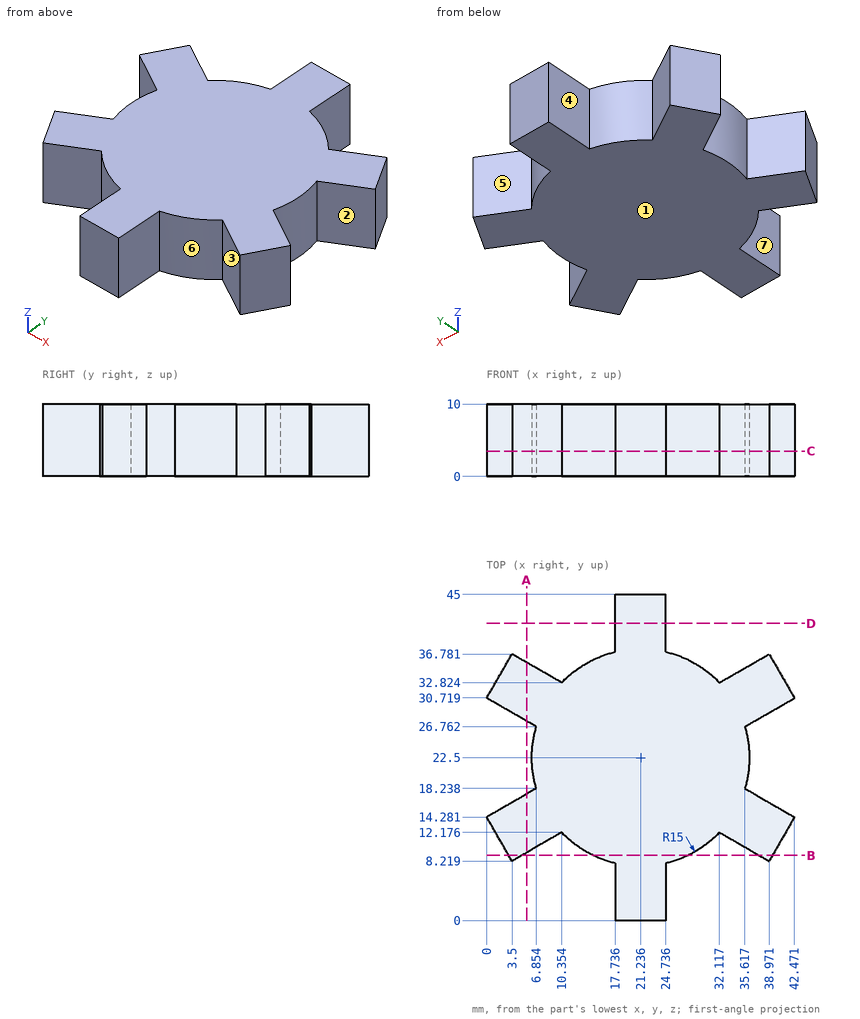
Job drawing, mm, ordinate dimensions from the low corner. One solid piece. A direction names the side the tool comes from. Coordinates: 2 decimals unless noted, no trailing zeros. Loops run counter-clockwise (first coordinate to the right, second up) from the corner with the lowest first, then second, coordinate; pieces in that order, holes last. Notation, with made-up numbers: (-17, 43.5) - (1, 43.5) arc R11 ccw to (1, 60.5) - close; hole circle Ø8 at (-2.5, -38.5). An arc over 180 degrees is marked (long way). Answer as a JSON object with one key per item and string values. Group by question number.
(1) Probe line 1 along X through (y, z) = (10, 0.5) (1 decimal); line 2 along X through (y, z) = (6, 3.75) (1 decimal); line 3 along Y through (x, z) = (4.5, 9.25) (1 decimal). List the from-to ranges inside material, lowest first.
(2) Flat gauge pins, fed straight in: pin 1 (6 mm diameter, centred on x = 32, z = 8.5, fed in from +Y) (1 decimal); pin 2 (4 mm diameter, centred on y = 40.5, z = 5.5, fed in from +X); pin 3 (3 mm diameter, centred on x = 6, z = 1, fed in from -Y); pin 4 (5 mm diameter, centred on x = 16, z = 5, fed in from +Y). Where does each tip first touch, or does it go through?
(3) Cut at B-B (y = 9). Give the cut face in (x, z), then the cut area to 3 significant figures.
(4) Tool access for the marked faces 5, 6 and 7: list every direction of +Z, -Z, +X, -X, +Y, -Y with a clear straight run to the whole face (end or side of a thin tool).
(5) Two-plate mould, pull along X, no slides. Class the marked faces 1, 2, 3 and 4: released by +X, released by -X, zero draft, split by the parting line, or undercut.
(6) Cut at C-C (z = 3.5). Give the cut face in (x, y) (1 decimal).
(7) Cut at D-D (y = 41). Give the cut face in (x, z) (1 decimal), then the cut area to 3 significant figures.
(8) Cut at A-A (x = 5.5). Give the cut face in (y, z).
Geometry says:
{
 "1": {"line 1": "x = 2.5 to 6.6, 12.9 to 29.5, 35.9 to 40", "line 2": "x = 17.7 to 24.7", "line 3": "y = 8.8 to 16.9, 28.1 to 36.2"},
 "2": {"pin 1": "stops at y = 35.3", "pin 2": "stops at x = 24.74", "pin 3": "stops at y = 8.8", "pin 4": "stops at y = 45"},
 "3": {"outline": "(3.05, 0) - (4.85, 0) - (4.85, 10) - (3.05, 10) - close; (14.7, 0) - (27.77, 0) - (27.77, 10) - (14.7, 10) - close; (37.62, 0) - (39.42, 0) - (39.42, 10) - (37.62, 10) - close", "area": "167 mm^2"},
 "4": {"face 5": "+Z, -Z, +Y", "face 6": "+Z, -Z, -Y", "face 7": "+Z, -Z, -X, -Y"},
 "5": {"face 1": "zero draft", "face 2": "released by +X", "face 3": "undercut", "face 4": "released by -X"},
 "6": {"outline": "(0, 14.3) - (3.5, 8.2) - (10.4, 12.2) arc R15 ccw to (17.7, 7.9) - (17.7, 0) - (24.7, 0) - (24.7, 7.9) arc R15 ccw to (32.1, 12.2) - (39, 8.2) - (42.5, 14.3) - (35.6, 18.2) arc R15 ccw to (35.6, 26.8) - (42.5, 30.7) - (39, 36.8) - (32.1, 32.8) arc R15 ccw to (24.7, 37.1) - (24.7, 45) - (17.7, 45) - (17.7, 37.1) arc R15 ccw to (10.4, 32.8) - (3.5, 36.8) - (0, 30.7) - (6.9, 26.8) arc R15 ccw to (6.9, 18.2) - close"},
 "7": {"outline": "(17.7, 0) - (24.7, 0) - (24.7, 10) - (17.7, 10) - close", "area": "70.0 mm^2"},
 "8": {"outline": "(9.37, 0) - (17.46, 0) - (17.46, 10) - (9.37, 10) - close; (27.54, 0) - (35.63, 0) - (35.63, 10) - (27.54, 10) - close"}
}
